Verification items for the finished model (mm, model axes). Face numbers are marked on the shaded views. Coordinates: 2 decimals unless noted, no trailing zeros. Write each loop counter-clockwise with the first axis right and the second up, starting at its lowest first coordinate (ties: lowest second). Pieces come first, ordered by that corner, then holes. Notation, with made-up numbers: M 80.5,38.5 L 107.5,38.5 A21 cw 107.5,44.5 Z; hole C -14.75,17 d3. An arc over 180 degrees is marked long. Answer in a Markdown table with one row per item.
Autodesk Inventor part; units mm, degrees
ref_plane "YZ Plane" through (0, 0, 0) normal (1, 0, 0) x (0, 1, 0)
ref_plane "XZ Plane" through (0, 0, 0) normal (0, 1, 0) x (-1, 0, 0)
ref_plane "XY Plane" through (0, 0, 0) normal (0, 0, 1) x (1, 0, 0)
sketch "Sketch1" plane through (0, 0, 0) normal (0, 1, 0) x (-1, 0, 0)
  circle A0 centre (0, 0) radius 12.5
  dimension "d0" = 25
extrude "Extrusion1" add sketch "Sketch1" along normal blind 52
sketch "Sketch2" plane through (0, 52, 0) normal (0, 1, 0) x (1, 0, 0)
  circle A0 centre (0, 0) radius 3.5
  dimension "d3" = 7
extrude "Extrusion2" add sketch "Sketch2" along normal blind 2
sketch "Sketch3" plane through (0, 54, 0) normal (0, 1, 0) x (1, 0, 0)
  circle A0 centre (0, 0) radius 2
  line L0 (-1.5, -2) -> (2, -2)
  line L1 (2, -2) -> (2, 2)
  line L2 (2, 2) -> (-1.5, 2)
  line L3 (-1.5, 2) -> (-1.5, -2)
  point P0 (-1.5, 1.3229)
  point P1 (-1.5, -1.3229)
  dimension "d6" = 4
  dimension "d7" = 3.5
extrude "Extrusion3" add sketch "Sketch3" along normal blind 10.7 contours A0 L3 picked at (0.1351, 0.5212)
sketch "Sketch4" plane through (0, 0, 0) normal (0, -1, 0) x (1, 0, 0)
  circle A0 centre (0, 0) radius 11.75
  dimension "d10" = 23.5
extrude "Extrusion4" cut sketch "Sketch4" against normal blind 1
sketch "Sketch5" plane through (0, 1, 0) normal (0, -1, 0) x (1, 0, 0)
  circle A0 centre (0, 0) radius 12.5
  circle A1 centre (0, 0) radius 3.25
  dimension "d13" = 6.5
extrude "Extrusion5" add sketch "Sketch5" along normal blind 2 contours A1
sketch "Sketch6" plane through (0, -1, 0) normal (0, -1, 0) x (1, 0, 0)
  circle A0 centre (0, 0) radius 1
  dimension "d16" = 2
extrude "Extrusion6" add sketch "Sketch6" along normal blind 6
sketch "Sketch7" plane through (0, 52, 0) normal (0, 1, 0) x (1, 0, 0)
  line L0 (0, 17.5) -> (0, -17.5)
  point P0 (0, 0)
  point P1 (-8.45, 0)
  point P2 (8.45, 0)
  dimension "d19" = 16.9
hole "Hole1" at (-8.45, 52, 0) at (8.45, 52, 0) direction (0, -1, 0) diameter 2.459 depth 8.8 tip angle 118
properties part number "Motor12V_V1" material "Steel"
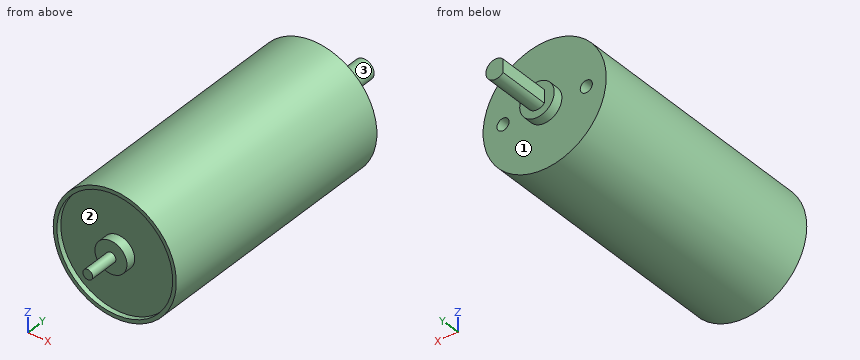
1) Depth check by flat-ended pin: pin 1 (4 mm diameter, centred on x = -8.45, z = 0, fed in from +Y); pin 2 (10 mm diameter, centred on y = 47, z = 6.5, fed in from +X); pin 3 (3 mm diameter, centred on x = -1, y = 56.5, fed in from +Z). Enter the tip coordinate at first touch or a pass-through.
Response values:
| item | result |
|---|---|
| pin 1 | stops at y = 52 |
| pin 2 | stops at x = 12.41 |
| pin 3 | stops at z = 2 |
2) Release check for a two-part mould opening along Z. For the marked faces 1, 2 and 3 record: +Z half, -Z half, draft (parallel to the pull), parting line (faces both ways), or undercut.
Response values:
| item | result |
|---|---|
| face 1 | draft |
| face 2 | undercut |
| face 3 | parting line |
3) Thickness scan on L1, parallel to Z at x = 0, y = 0.8; L2, parallel to Y at x = 9.75, z = -6.25; L3, parallel to Y at x = 0.5, z = -1.5. Record the ranges inside material, lowest first. Write a range as [from, to].
Response values:
| item | result |
|---|---|
| L1 | z = [-12.5, -11.75], [-3.25, 3.25], [11.75, 12.5] |
| L2 | y = [1, 52] |
| L3 | y = [-1, 64.7] |
4) Sectioned sample at A-A (x = 0). Record the cut outline in (y, z), then the cut area to 3 significant figures.
Response values:
| item | result |
|---|---|
| outline | M -7,-1 L -1,-1 L -1,-3.25 L 1,-3.25 L 1,-11.75 L 0,-11.75 L 0,-12.5 L 52,-12.5 L 52,-3.5 L 54,-3.5 L 54,-2 L 64.7,-2 L 64.7,2 L 54,2 L 54,3.5 L 52,3.5 L 52,12.5 L 0,12.5 L 0,11.75 L 1,11.75 L 1,3.25 L -1,3.25 L -1,1 L -7,1 Z |
| area | 1,360 mm² |
5) Sectioned sample at C-C (z = 6.5). Record the cut outline in (x, y).
Response values:
| item | result |
|---|---|
| outline | M -10.68,0 L -9.79,0 L -9.79,1 L 9.79,1 L 9.79,0 L 10.68,0 L 10.68,52 L -10.68,52 Z |
6) Sectioned sample at B-B (z = 9.5). Record the cut outline in (x, y).
Response values:
| item | result |
|---|---|
| outline | M -8.12,0 L -6.91,0 L -6.91,1 L 6.91,1 L 6.91,0 L 8.12,0 L 8.12,52 L -8.12,52 Z |
